Verification items for this drawing (mm, ordinates from the low corner). Round coordinates to 2 decimals unless told otherwise and drop trailing zeros. Order: outer loops, then holes, each group sorted by start corner. A loop starts at its lowest first (then second) coordinate and runs counter-clockwise, first axis right, second up. Notation, with made-up numbers: (-38.5, -26.5) -> (15.5, -26.5) arc R33 cw to (15.5, 1.5) -> close; hole circle Ø2 at (40.25, 39.5). An arc over 180 degrees is marked (long way). Answer in a Markdown table with one row per item.
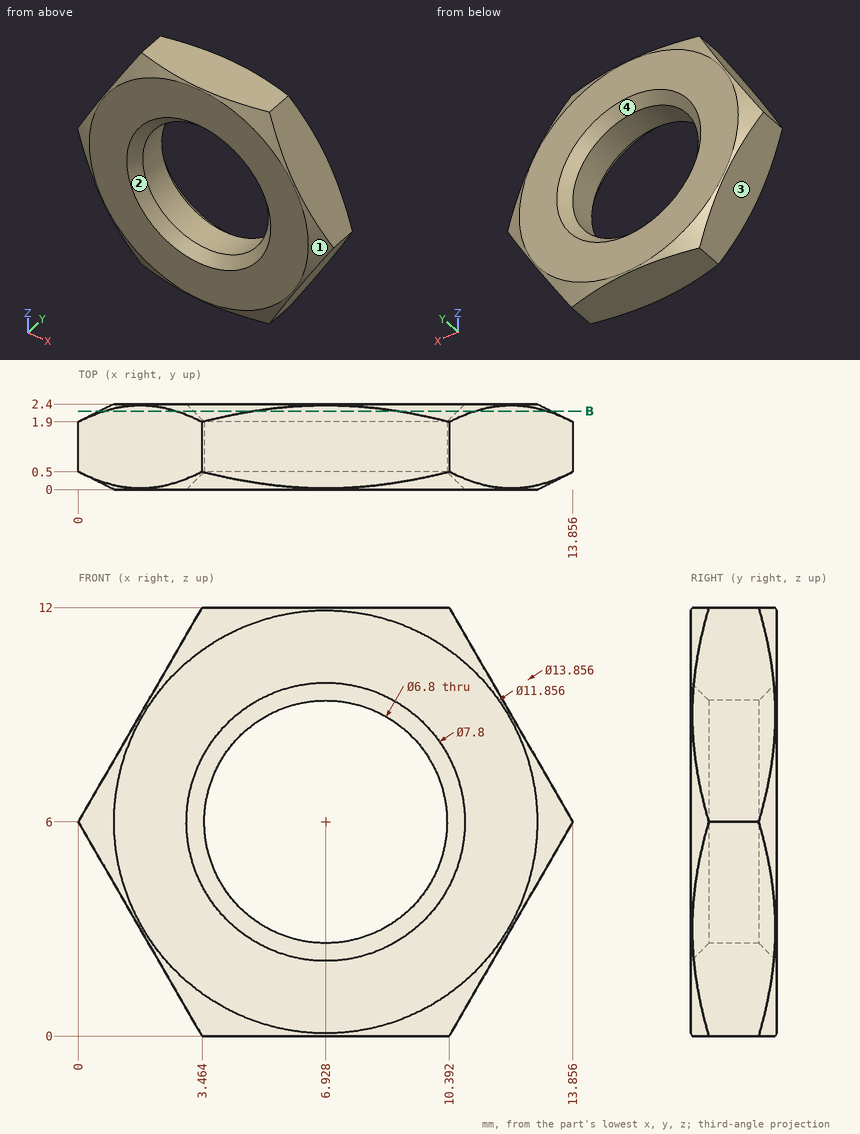
Item 1: Cross-section at B-B (y = 2.2). Record the boundary of the cut face in (x, z).
Result sheet:
| item | result |
|---|---|
| outline | (0.73, 4.74) -> (2.74, 1.26) arc R6.33 ccw to (4.92, 0) -> (8.94, 0) arc R6.33 ccw to (11.12, 1.26) -> (13.13, 4.74) arc R6.33 ccw to (13.13, 7.26) -> (11.12, 10.74) arc R6.33 ccw to (8.94, 12) -> (4.92, 12) arc R6.33 ccw to (2.74, 10.74) -> (0.73, 7.26) arc R6.33 ccw to start; hole circle Ø7.4 at (6.93, 6) |
Item 2: Mould release check, pull along Z, two halves, no side actions. Record for the marked faces 1, 2, 3 and 4: pulls with the +Z half, pulls with the -Z half, needs draft (parallel to the pull), parting line crosses it, or undercut.
Result sheet:
| item | result |
|---|---|
| face 1 | parting line crosses it |
| face 2 | undercut |
| face 3 | pulls with the -Z half |
| face 4 | undercut |
Item 3: Scan lines: line 1 (X direction, y = 1.95, z = 5.25) (1 decimal); line 2 (X direction, y = 0.9, z = 3.5) (1 decimal); line 3 (Z direction, x = 2.25, y = 0.7) (1 decimal). Record each from-to range of solid material in increasing order. Write a range as [from, to].
Result sheet:
| item | result |
|---|---|
| line 1 | x = [0.4, 3.6], [10.3, 13.4] |
| line 2 | x = [1.4, 4.6], [9.2, 12.4] |
| line 3 | z = [2.1, 9.9] |
Item 4: Depth check by flat-ended pin: P1, Ø1, axis at y = 0.5, z = 3.5, coming from the +X side. Enter the tip coordinate at first touch or a pass-through.
Result sheet:
| item | result |
|---|---|
| P1 | stops at x = 12.7 |
